The model under review builds one solid part; all positions refer to its coordinate system, in mm. Round coordinates to 2 decimals unless told otherwise and drop trailing zeros. Write each loop counter-clockwise with the first axis right and the second up, starting at its lowest first coordinate (ties: lowest second). Pieces come first, ordered by that corner, then holes. Notation, with made-up numbers: (73, 78.25) -> (123, 78.25) arc R25 ccw to (123, 117.25) -> close; hole circle Ø9 at (39.25, -29). An arc over 180 degrees is marked (long way). Answer in a Markdown table with one row per item. Add a question column.
```python
from build123d import *

# Parameters (mm, degrees)
SCHIZZO1_R                   = 6
ESTRUSIONE_ESTRUSIONE1_DEPTH = 112.5


with BuildPart() as part:
    # Schizzo1 → Estrusione-Estrusione1 (new, symmetric)
    with BuildSketch(Plane.XY):
        Circle(SCHIZZO1_R)
    extrude(amount=ESTRUSIONE_ESTRUSIONE1_DEPTH, both=True)

    # Schizzo3 → Foro per Vite M6-1 (revolve, cut)
    with BuildSketch(Plane(origin=(0, 0, 112.5), x_dir=(0, -1, 0), z_dir=(1, 0, 0))):
        Polygon((0, 0), (0, 25), (3.2, 23.077246019), (3.2, 0), align=None)
    foro_per_vite_m6_1 = revolve(axis=Axis((0, 0, 118.85), (0, 0, -1)), mode=Mode.SUBTRACT)

    # Specchia1: Foro per Vite M6-1 across plane
    add(foro_per_vite_m6_1.mirror(Plane.XY), mode=Mode.SUBTRACT)


solid = part.part
```
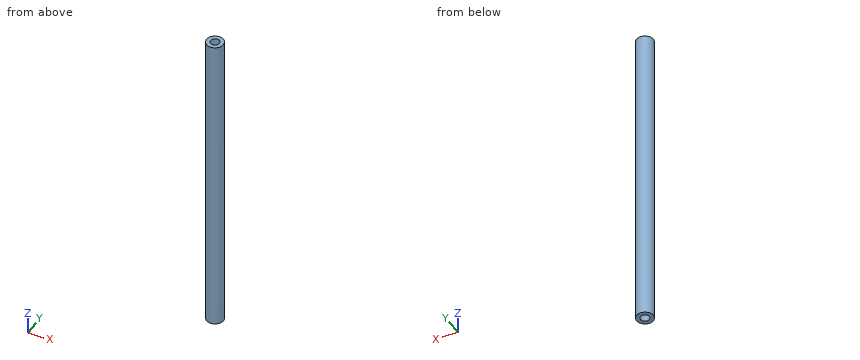
1. Add section A-A on z = -72. Write out the cut boundary in (x, y), plus the area to 3 significant figures.
2. For L1, parallel to Y at x = 0, z = -101; L2, parallel to X at y = -1.5, z = -90.5; L3, parallel to X at y = -1.75, z = 96.5, list the stretches that pass through material, from the lowest coordinate up.
3. Insertion check: pin 1 Ø5 at (x, y) = (0.5, -1.5) entering from -Z; pin 2 Ø5 at (x, z) = (4, -53) entering from -Y; pin 3 Ø6 at (x, y) = (0, 0) entering from +Z; pin 4 Ø2 at (x, y) = (2, 0) entering from -Z. Each pin has a flat end and moves straight along its axis. Give the tip position at first contact, or say it passes through.
Filled in:
| question | item | result |
|---|---|---|
| 1 | outline | circle Ø12 at (0, 0) |
| 1 | area | 113 mm² |
| 2 | L1 | -6 to -3.2, 3.2 to 6 |
| 2 | L2 | -5.81 to -2.83, 2.83 to 5.81 |
| 2 | L3 | -5.74 to -2.68, 2.68 to 5.74 |
| 3 | pin 1 | z = -112.5 |
| 3 | pin 2 | y = -5.81 |
| 3 | pin 3 | z = 89.3 |
| 3 | pin 4 | z = -89.3 |
